Answer from the drawing. Dimensions are ordinates in mm from the lowest x, y and z of the part. Coordinates: 2 decimals unless noted, no trailing zeros. Write each loop counter-clockwise with the first axis right and the second up, starting at its lowest first coordinate (ties: lowest second). Pieces come first, ordered by that corner, then holes. Notation, with made-up numbers: (80.5, 82) -> (134.5, 82) arc R18 ccw to (134.5, 94) -> close; hole circle Ø7 at (16, -28.75). An arc over 180 degrees is marked (long way). Answer as a JSON object with one key per item and string values. Group by question number.
(1) Find section C-C (x = 97). Give the vertices of the cut face in (y, z).
(2) Find section A-A (z = 97). Give the vertices of the cut face in (x, y).
(3) Straight lines are drawn through the part: L1, parallel to Z at x = 99, y = 0.75; L2, parallel to Z at x = 184, y = 8.1. For each, find the intervals that lie inside material, in ascending order.
(4) Flat-ended cylindrical pins translate along their axes: P1, Ø7, axis at x = 184, z = 97, coming from the -Y side; P2, Ø6, axis at x = 46, y = 6.5, coming from the -Z side; P3, Ø6, axis at y = 7.5, z = 48, coming from the -X side; P4, Ø5.5, axis at x = 97, z = 184, coming from the +Y side. Find the tip coordinate at first contact, or state that the pin passes through.
(5) Find section B-B (y = 6.25). Give the vertices of the cut face in (x, z).
(6) Find section D-D (x = 10). Give the vertices of the cut face in (y, z).
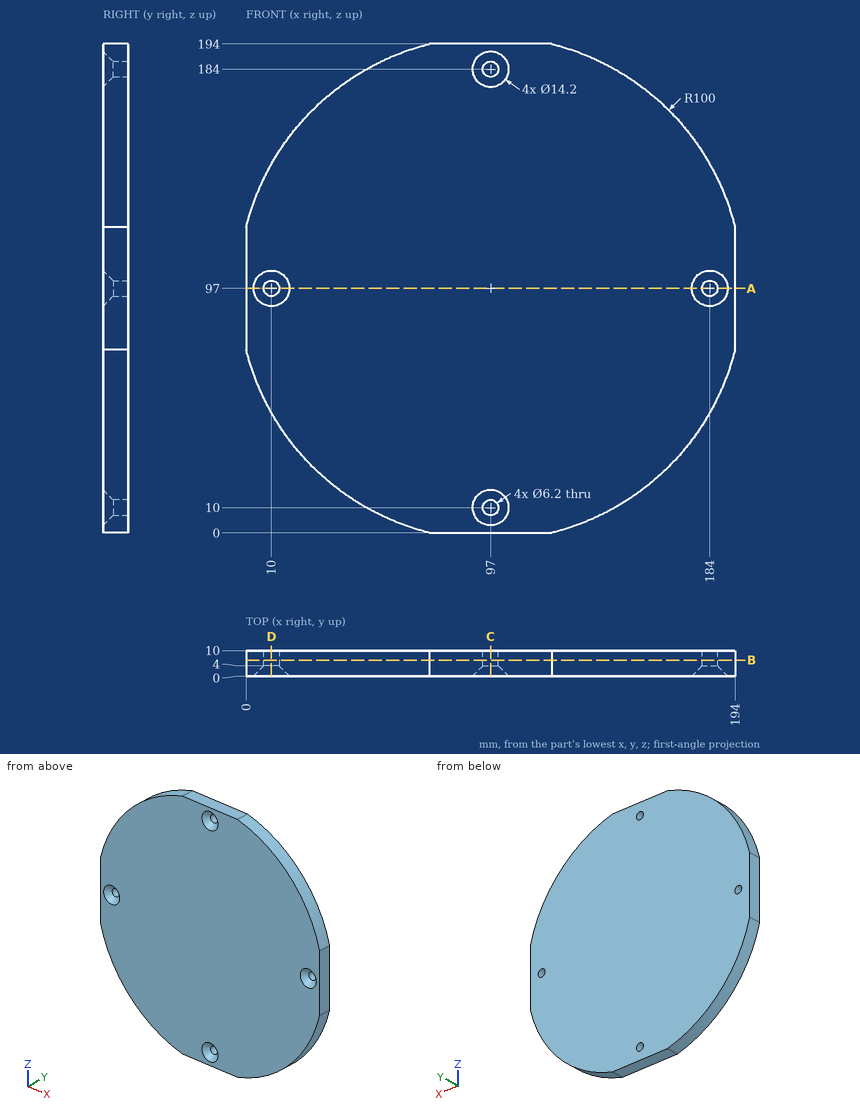
Results below:
{
 "1": {"outline": "(0, 0) -> (10, 0) -> (10, 6.9) -> (4, 6.9) -> (0, 2.9) -> close; (0, 17.1) -> (4, 13.1) -> (10, 13.1) -> (10, 180.9) -> (4, 180.9) -> (0, 176.9) -> close; (0, 191.1) -> (4, 187.1) -> (10, 187.1) -> (10, 194) -> (0, 194) -> close"},
 "2": {"outline": "(0, 0) -> (2.9, 0) -> (6.9, 4) -> (6.9, 10) -> (0, 10) -> close; (13.1, 4) -> (17.1, 0) -> (176.9, 0) -> (180.9, 4) -> (180.9, 10) -> (13.1, 10) -> close; (187.1, 4) -> (191.1, 0) -> (194, 0) -> (194, 10) -> (187.1, 10) -> close"},
 "3": {"L1": "z = 0 to 3.97, 16.03 to 177.97, 190.03 to 194", "L2": "z = 47.69 to 93.9, 100.1 to 146.31"},
 "4": {"P1": "stops at y = 3.6", "P2": "stops at z = 9.27", "P3": "stops at x = 8.21", "P4": "passes through"},
 "5": {"outline": "(0, 72.69) arc R100 ccw to (72.69, 0) -> (121.31, 0) arc R100 ccw to (194, 72.69) -> (194, 121.31) arc R100 ccw to (121.31, 194) -> (72.69, 194) arc R100 ccw to (0, 121.31) -> close; hole circle Ø6.2 at (10, 97); hole circle Ø6.2 at (97, 10); hole circle Ø6.2 at (97, 184); hole circle Ø6.2 at (184, 97)"},
 "6": {"outline": "(0, 47.69) -> (10, 47.69) -> (10, 93.9) -> (4, 93.9) -> (0, 89.9) -> close; (0, 104.1) -> (4, 100.1) -> (10, 100.1) -> (10, 146.31) -> (0, 146.31) -> close"}
}
